Part model, mm, in its own coordinate system. Round coordinates to 2 decimals unless told otherwise and drop trailing zeros. Write each loop counter-clockwise with the first axis right and the second up, starting at its lowest first coordinate (ties: lowest second). Pieces come first, ordered by that corner, then holes. Notation, with made-up numbers: M -18,43.25 L 9,43.25 A20 ccw 9,66.25 Z; hole C 10,-15.5 d9. An arc over 180 degrees is marked long. Use one line per item in the form item = value. Start each with the question number.
Item 1: Probe L1, parallel to X at y = 507, z = -15; L2, parallel to X at y = 322.5, z = -8.75; L3, parallel to X at y = 323, z = -1. List the from-to ranges inside material, lowest first.
Item 2: Cut at C-C, the plane y = 218.5. Give the cut face in (x, z).
Item 3: Cut at B-B, the plane z = -16. State how many separate pieces and enclosed holes the cut face has, then the cut area to 3 significant figures.
Item 4: Cut at A-A, the plane x = -537. Give the cut face in (y, z).
Item 5: Flat gauge pins, fed straight in: pin 1 Ø3 at (x, y) = (-345.07, 437.89) entering from -Z; pin 2 Ø5 at (y, z) = (277, -2) entering from +X; pin 3 Ø1.5 at (y, z) = (242, -4) entering from -X (3 decimals); pin 4 Ø3 at (x, z) = (-546.5, -7.5) entering from +Y. Where does each tip first touch, or does it go through?
from build123d import *

# Parameters (mm, degrees)
BOSS_EXTRUDE1_DEPTH        = 19.05
BOSS_EXTRUDE2_DEPTH        = 19.05
FILLET1_R                  = 3.175
FILLET2_R                  = 12.7
SKETCH47_R                 = 3.175
CUT_EXTRUDE1_DEPTH         = 1
CUT_EXTRUDE1_DEPTH_BACK    = 20.05
FILLET4_R                  = 6.35
F_1_2_0_5_DIAMETER_HOLE1_D = 12.7
HOLE7_D                    = 3.175
HOLE7_DEPTH                = 38.1
HOLE7_CSINK_D              = 10.16
HOLE7_CSINK_ANGLE          = 82
HOLE7_TIP                  = 0.953866233
HOLE10_D                   = 3.175
HOLE10_DEPTH               = 57.15
HOLE10_CSINK_D             = 10.16
HOLE10_CSINK_ANGLE         = 82
HOLE10_TIP                 = 0.953866233
HOLE13_D                   = 3.175
HOLE13_DEPTH               = 31.75
HOLE13_CSINK_D             = 10.16
HOLE13_CSINK_ANGLE         = 82
HOLE13_TIP                 = 0.953866233


with BuildPart() as part:
    # Sketch1 → Boss-Extrude1 (new body)
    with BuildSketch(Plane.XY):
        Polygon((-247.274665566, 82.142339986), (-381.523973725, 38.103910865), (-614.640105377, 748.748682245), (-504.525442447, 784.870110692), (-417.251419261, 518.818903446), (-393.116774032, 526.735904121), align=None)
    extrude(amount=-BOSS_EXTRUDE1_DEPTH)

    # Sketch2 → Boss-Extrude2 (add, through all)
    with BuildSketch(Plane.XY):
        Polygon((-393.116774032, 526.735904121), (-336.901176267, 355.36500697), (-277.604402796, 374.816405204), (-281.415155825, 417.005352091), (-320.44916939, 493.083731154), (-290.280862854, 502.979981998), (-307.307307279, 554.884385267), align=None)
    extrude(amount=-BOSS_EXTRUDE2_DEPTH)

    # Fillet1
    fillet1_edges = [part.edges().sort_by_distance(p)[0] for p in [
        (-320.44916939, 493.083731154, -9.525),
    ]]
    fillet(fillet1_edges, radius=FILLET1_R)

    # Fillet2
    fillet2_edges = [part.edges().sort_by_distance(p)[0] for p in [
        (-336.901176267, 355.36500697, -9.525),
    ]]
    fillet(fillet2_edges, radius=FILLET2_R)

    # Sketch47 → Cut-Extrude1 (cut, two sides)
    with BuildSketch(Plane(origin=(0, 0, -19.05), x_dir=(-1, 0, 0), z_dir=(0, 0, -1))) as cut_extrude1_sk:
        with Locations((417.251419261, 518.818903446)):
            Circle(SKETCH47_R)
    extrude(amount=CUT_EXTRUDE1_DEPTH, mode=Mode.SUBTRACT)
    extrude(cut_extrude1_sk.sketch, amount=-CUT_EXTRUDE1_DEPTH_BACK, mode=Mode.SUBTRACT)

    # Fillet4
    fillet4_edges = [part.edges().sort_by_distance(p)[0] for p in [
        (-418.241044345, 521.8357341, -9.525),
        (-414.234588607, 519.80852853, -9.525),
    ]]
    fillet(fillet4_edges, radius=FILLET4_R)

    # 1/2 (0.5) Diameter Hole1 (through all)
    with Locations(Plane.XY):
        with Locations((-563.45033927, 698.544682362), (-504.072834209, 517.534843147), (-316.771364786, 371.99266929), (-323.698740376, 393.110483865), (-289.824308357, 404.222472403), (-287.772364418, 381.505347156), (-305.715281117, 417.978415836), (-364.985283482, 398.535799453), (-384.427899865, 457.805801818), (-325.157897499, 477.248418201), (-332.468536604, 499.165347862), (-305.317060721, 508.071973621), (-316.40575464, 541.875392969), (-343.557230523, 532.968767209)):
            Hole(F_1_2_0_5_DIAMETER_HOLE1_D / 2)

    # Hole7
    with Locations(Plane(origin=(313.774034821, -375.700785936, 19.05), x_dir=(0.997756458, -0.066948111, 0), z_dir=(0, 0, 1))):
        with Locations((-710.914924699, 391.126528253), (-615.24080496, 429.781381762), (-711.83598555, 767.659094962), (-835.937309391, 717.51890547), (-904.68821492, 1078.38439498), (-976.811864753, 1049.244548945)):
            CounterSinkHole(HOLE7_D / 2, HOLE7_CSINK_D / 2, depth=HOLE7_DEPTH, counter_sink_angle=HOLE7_CSINK_ANGLE)
            with Locations((0, 0, -(HOLE7_DEPTH + HOLE7_TIP / 2))):  # 118° drill point
                Cone(0, HOLE7_D / 2, HOLE7_TIP, mode=Mode.SUBTRACT)

    # Hole10
    with Locations(Plane(origin=(313.774034821, -375.700785936, -57.15), x_dir=(-0.997756458, 0.066948111, 0), z_dir=(0, 0, -1))):
        with Locations((848.944412528, 940.413642522), (885.927448463, 1031.949868564), (867.435930496, 986.181755543), (830.452894561, 894.645529501)):
            CounterSinkHole(HOLE10_D / 2, HOLE10_CSINK_D / 2, depth=HOLE10_DEPTH, counter_sink_angle=HOLE10_CSINK_ANGLE)
            with Locations((0, 0, -(HOLE10_DEPTH + HOLE10_TIP / 2))):  # 118° drill point
                Cone(0, HOLE10_D / 2, HOLE10_TIP, mode=Mode.SUBTRACT)

    # Hole13
    with Locations(Plane(origin=(-45.102820315, -493.424841017, 52.974999997), x_dir=(0, 0, -1), z_dir=(0.950182883, 0.31169294, 0))):
        with Locations((174.999999994, 685.961004241), (174.999999994, 549.837259632), (174.999999994, 413.713515022), (81.549999997, 779.649723129), (81.549999997, 652.344645962), (62.499999997, 662.953402392), (62.499999997, 769.040966698), (-62.499999997, 769.040966698), (-62.499999997, 662.953402392), (-81.549999997, 652.344645962), (-81.549999997, 779.649723129), (-174.999999994, 413.713515022), (-174.999999994, 549.837259632), (-174.999999994, 685.961004241), (-82.737499997, 600.384620239), (0, 600.384620239), (82.737499997, 600.384620239), (0, 376.737770337), (-82.737499997, 376.737770337), (82.737499997, 376.737770337)):
            CounterSinkHole(HOLE13_D / 2, HOLE13_CSINK_D / 2, depth=HOLE13_DEPTH, counter_sink_angle=HOLE13_CSINK_ANGLE)
            with Locations((0, 0, -(HOLE13_DEPTH + HOLE13_TIP / 2))):  # 118° drill point
                Cone(0, HOLE13_D / 2, HOLE13_TIP, mode=Mode.SUBTRACT)


solid = part.part
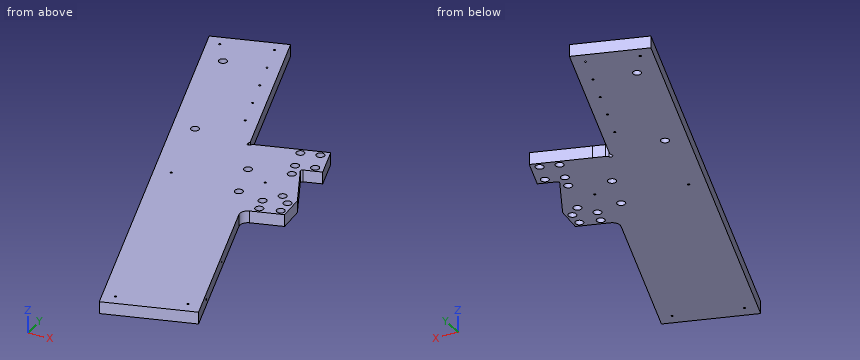
Model answer:
q1.L1 = -535.34 to -311.58, -299.06 to -291.6
q1.L2 = -474.82 to -326.12
q1.L3 = -474.98 to -326.28
q2.outline = M -440.7,-19.05 L -292,-19.05 L -292,0 L -440.7,0 Z
q3.separate_pieces = 1
q3.enclosed_holes = 24
q3.area = 110,000 mm²
q4.outline = M 512.07,-19.05 L 774.22,-19.05 L 774.22,0 L 512.07,0 Z
q5.pin_1 = through
q5.pin_2 = -310.37
q5.pin_3 = -448.655
q5.pin_4 = 771.59
